from build123d import *

# Parameters (mm, degrees)
SKETCH1_R           = 1.75
SKETCH1_R_2         = 5.25
BOSS_EXTRUDE1_DEPTH = 10
EXTRUDE1_DEPTH      = 5
FILLET2_R           = 20
FILLET3_R           = 5
FILLET5_R           = 5
EXTRUDE2_DEPTH      = 5
FILLET7_R           = 475
FILLET8_R           = 15
FILLET9_R           = 5
SKETCH4_R           = 3.5
EXTRUDE3_DEPTH      = 2


with BuildPart() as part:
    # Sketch1 → Boss-Extrude1 (new body)
    with BuildSketch(Plane.XY):
        with BuildLine():
            Line((59.115327383, 43.551262968), (59.822811009, 43.551262968))
            ThreePointArc((59.822811009, 43.551262968), (62.822811009, 44.551262968), (65.822811009, 43.551262968))
            Line((65.822811009, 43.551262968), (90.822811009, 43.551262968))
            ThreePointArc((90.822811009, 43.551262968), (98.822811009, 39.551262968), (90.822811009, 35.551262968))
            Line((90.822811009, 35.551262968), (73.221068218, 35.551262968))
            ThreePointArc((73.221068218, 35.551262968), (65.430500205, 30.870379763), (65.905746743, 21.794160382))
            add(Edge.make_bspline(
                [(65.905746743, 21.794160382), (68.510586107, 17.931817085), (68.397648351, 12.955422289), (67.785956814, 7.945306105)],
                knots=[0, 0, 0, 0, 1, 1, 1, 1], degree=3))
            ThreePointArc((67.785956814, 7.945306105), (67.117243875, 5.990433735), (65.715264602, 4.47281814))
            ThreePointArc((65.715264602, 4.47281814), (62.263505272, 3.582643734), (59.096031047, 5.217929635))
            ThreePointArc((59.096031047, 5.217929635), (55.724954026, 7.67997226), (51.642471122, 8.551262968))
            Line((51.642471122, 8.551262968), (46.826949913, 8.551262968))
            ThreePointArc((46.826949913, 8.551262968), (39.614460745, 11.5387738), (36.626949913, 18.751262968))
            Line((36.626949913, 18.751262968), (36.626949913, 38.848632096))
            ThreePointArc((36.626949913, 38.848632096), (42.251881835, 47.568318218), (52.515088487, 46.03881686))
            ThreePointArc((52.515088487, 46.03881686), (55.588605185, 44.19379373), (59.115327383, 43.551262968))
        make_face()
        with Locations((93.822811009, 39.551262968)):
            Circle(SKETCH1_R, mode=Mode.SUBTRACT)
        with Locations((62.822811009, 39.551262968)):
            Circle(SKETCH1_R, mode=Mode.SUBTRACT)
        with Locations((62.822811009, 8.551262968)):
            Circle(SKETCH1_R, mode=Mode.SUBTRACT)
        with Locations((45.725055781, 39.551262968)):
            Circle(SKETCH1_R_2, mode=Mode.SUBTRACT)
        with Locations((45.725055781, 17.551264875)):
            Circle(SKETCH1_R_2, mode=Mode.SUBTRACT)
    extrude(amount=-BOSS_EXTRUDE1_DEPTH)

    # Sketch2 → Extrude1 (add)
    with BuildSketch(Plane.XY):
        Polygon((45.636633265, 8.551262968), (43.896905309, -1.448737032), (10.896905309, -1.448737032), (10.896905309, 16.551262968), (37.366610934, 16.551262968), (39.363957543, 12.249932276), (45.636633265, 10.857586925), align=None)
    extrude(amount=-EXTRUDE1_DEPTH)

    # Fillet2
    # the kernel refuses this fillet: 20 mm, written as the material it adds along each edge
    with BuildSketch(Plane(origin=(36.867030235, 16.551262968, -5), x_dir=(-0.0120031513061412, 0.9999279595844501, 0), z_dir=(0, 0, 1))) as fillet2_piece_1:
        with BuildLine():
            CenterArc((20.241503938, 19.998559192), FILLET2_R, 179.312253574, 90)
            Line((0.242944747, 20.238622218), (-1.756911173, 20.26262852))
            Line((-1.756911173, 20.26262852), (-1.999855919, 0.024006303))
            Line((-1.999855919, 0.024006303), (0.407900213, -1.957962568))
            ThreePointArc((0.407900213, -1.957962568), (2.178716929, -1.786199826), (19.97743461, -1.999855919))
            Line((19.97743461, -1.999855919), (20.001440912, 0))
        make_face()
    extrude(amount=5)

    # Fillet3
    fillet3_edges = [part.edges().sort_by_distance(p)[0] for p in [
        (10.896905309, 16.551262968, -2.5),
    ]]
    fillet(fillet3_edges, radius=FILLET3_R)

    # Fillet5
    fillet5_edges = [part.edges().sort_by_distance(p)[0] for p in [
        (10.896905309, -1.448737032, -2.5),
    ]]
    fillet(fillet5_edges, radius=FILLET5_R)

    # Sketch3 → Extrude2 (cut)
    with BuildSketch(Plane(origin=(0, 0, -5), x_dir=(-1, 0, 0), z_dir=(0, 0, -1))):
        with BuildLine():
            Line((-15.230767467, 10.918134064), (-35.230767467, 10.918134064))
            ThreePointArc((-35.230767467, 10.918134064), (-36.730767467, 12.418134064), (-35.230767467, 13.918134064))
            Line((-35.230767467, 13.918134064), (-15.230767467, 13.918134064))
            ThreePointArc((-15.230767467, 13.918134064), (-13.730767467, 12.418134064), (-15.230767467, 10.918134064))
        make_face()
        with BuildLine():
            Line((-15.725055781, 2.918134064), (-40.725055781, 2.918134064))
            ThreePointArc((-40.725055781, 2.918134064), (-42.225055781, 4.418134064), (-40.725055781, 5.918134064))
            Line((-40.725055781, 5.918134064), (-15.725055781, 5.918134064))
            ThreePointArc((-15.725055781, 5.918134064), (-14.225055781, 4.418134064), (-15.725055781, 2.918134064))
        make_face()
    extrude(amount=-EXTRUDE2_DEPTH, mode=Mode.SUBTRACT)

    # Fillet7
    # the kernel refuses this fillet: 475 mm, written as the material it adds along each edge
    with BuildSketch(Plane(origin=(45.636633265, 8.620954667, -5), x_dir=(0, -1, 0), z_dir=(0, 0, 1))) as fillet7_piece_1:
        with BuildLine():
            CenterArc((475.069322793, 0.591997114), FILLET7_R, 179.929346264, 0.142062041)
            ThreePointArc((0.069683944, 1.17773862), (0.051884348, 0.587860954), (0, 0))
            Line((0, 0), (0.069691699, 0))
        make_face()
    extrude(amount=5)

    # Fillet8
    # the kernel refuses this fillet: 15 mm, written as the material it adds along each edge
    with BuildSketch(Plane(origin=(45.636633265, 8.551262968, 0), x_dir=(0.9999999999783198, 6.584854434625016e-06, 0), z_dir=(0, 0, -1))) as fillet8_piece_1:
        with BuildLine():
            CenterArc((13.821083543, 8.071296621), FILLET8_R, 189.869507231, 22.683962159)
            Line((-0.956926764, 5.500224598), (0, 0))
            ThreePointArc((0, 0), (0.58886931, -0.000365018), (1.17773862, 0))
        make_face()
    extrude(amount=5)

    # Fillet9
    fillet9_edges = [part.edges().sort_by_distance(p)[0] for p in [
        (43.896905309, -1.448737032, -2.5),
    ]]
    fillet(fillet9_edges, radius=FILLET9_R)

    # Sketch4 → Extrude3 (cut)
    with BuildSketch(Plane(origin=(0, 0, -10), x_dir=(-1, 0, 0), z_dir=(0, 0, -1))):
        with Locations((-62.822811009, 39.551262968)):
            Circle(SKETCH4_R)
        with Locations((-93.822811009, 39.551262968)):
            Circle(SKETCH4_R)
        with Locations((-62.822811009, 8.551262968)):
            Circle(SKETCH4_R)
    extrude(amount=-EXTRUDE3_DEPTH, mode=Mode.SUBTRACT)


solid = part.part
The listing builds one solid part. Answer for the finished solid, in the listing's coordinates (mm). A direction names the side the tool comes from. Coordinates: 2 decimals unless noted, no trailing zeros. Write each loop counter-clockwise with the first axis right and the second up, starting at its lowest first coordinate (ties: lowest second). Pieces come first, ordered by that corner, then holes. Notation, with made-up numbers: (33, 41.5) -> (77, 41.5) arc R8 cw to (77, 46.5) -> close; hole circle Ø10 at (-6.5, 40). An arc over 180 degrees is marked (long way). One line per question, with ' | ' between items.
1. Straight lines are drawn through the part: line 1 (Z direction, x = 33, y = 21); line 2 (Y direction, x = 19.5, z = -3.75); line 3 (Y direction, x = 34.5, z = -1.5). For each, find the intervals that lie inside material, in ascending order.
Verdict:
line 1: z = -5 to 0 | line 2: y = -1.45 to 2.92, 5.92 to 10.92, 13.92 to 16.76 | line 3: y = -1.45 to 2.92, 5.92 to 10.92, 13.92 to 27.58
2. Section D-D (y = 25.5) is taken. Determine the outline of the cut face in (x, z).
Verdict:
outline: (33.3, -5) -> (36.63, -5) -> (36.63, -10) -> (64.48, -10) -> (64.48, 0) -> (33.3, 0) -> close
3. Given pin 1 Ø3 at (y, z) = (30, -7) entering from -X; pin 2 Ø1.5 at (x, z) = (24.5, -1.5) entering from +Y; pin 3 Ø10 at (x, y) = (22, 24) entering from +Z; pin 4 Ø2 at (x, y) = (64, 9.5) entering from -Z, each flat-ended and moving along its own axis, determine where each tip first touches the part or whether it passes through.
Verdict:
pin 1: stops at x = 36.63 | pin 2: stops at y = 18.51 | pin 3: passes through | pin 4: stops at z = -8
4. For a pull along X with two mould halves and no side action, classify faces 6 (the flat face through (28, -1.449, -2)), 7 (the cylindrical face through (30.61, 22.25, -2.54)), 8 (the cylindrical face through (62.443, 37.843, -3.944)) as released by +X, released by -X, zero draft, split by the parting line, or undercut.
Verdict:
face 6: zero draft | face 7: released by -X | face 8: undercut
5. Section B-B (x = 62.5) is taken. Determine the outline of the cut face in (y, z), and give its area (3 significant figures).
Verdict:
outline: (3.56, -10) -> (5.07, -10) -> (5.07, -8) -> (6.83, -8) -> (6.83, 0) -> (3.56, 0) -> close; (10.27, -8) -> (12.04, -8) -> (12.04, -10) -> (36.07, -10) -> (36.07, -8) -> (37.83, -8) -> (37.83, 0) -> (10.27, 0) -> close; (41.27, -8) -> (43.04, -8) -> (43.04, -10) -> (44.54, -10) -> (44.54, 0) -> (41.27, 0) -> close | area: 327 mm^2
6. Which of the six approach directions +Z, -Z, +X, -X, +Y, -Y give full straight-line access (tool end or side, diameter ignored) to faces 1 (the cylindrical face through (55.541, 44.212, -4.93)), 2 (the flat face through (61, 7, -8)), 3 (the flat face through (28, 2.918, -3)), 4 (the cylindrical face through (45.46, 5.87, -2.46)), 5 (the flat face through (52, 23, 0))?
Verdict:
face 1: +Z, -Z, +Y | face 2: -Z | face 3: +Z, -Z | face 4: +Z, -Z, -Y | face 5: +Z, +X, -X, +Y, -Y
7. Section A-A (x = 20.5) is taken. Determine the outline of the cut face in (y, z), and give its area (3 significant figures).
Verdict:
outline: (-1.45, -5) -> (2.92, -5) -> (2.92, 0) -> (-1.45, 0) -> close; (5.92, -5) -> (10.92, -5) -> (10.92, 0) -> (5.92, 0) -> close; (13.92, -5) -> (16.93, -5) -> (16.93, 0) -> (13.92, 0) -> close | area: 61.9 mm^2
8. Section C-C (z = -6.25) is taken. State how many separate pieces and enclosed holes the cut face has, and give its area (3 significant figures).
Verdict:
separate pieces: 1 | enclosed holes: 5 | area: 1,200 mm^2
